Geometry check sheet. Reference: the model listing, model coordinates, mm. Round coordinates to 2 decimals unless told otherwise and drop trailing zeros. Write each loop counter-clockwise with the first axis right and the second up, starting at its lowest first coordinate (ties: lowest second). Pieces come first, ordered by that corner, then holes. Notation, with made-up numbers: (59.25, 6.25) - (92.25, 6.25) arc R21 ccw to (92.25, 32.25) - close; hole circle Ø4 at (15.5, 60). An arc over 180 degrees is marked (long way). Return JSON: item names as keys, results as strings.
```python
from build123d import *

# Parameters (mm, degrees)
SKETCH1_W           = 104
SKETCH1_H           = 104
SKETCH1_W_2         = 100
SKETCH1_H_2         = 100
BOSS_EXTRUDE1_DEPTH = 2


with BuildPart() as part:
    # Sketch1 → Boss-Extrude1 (new body)
    with BuildSketch(Plane(origin=(0, 0, 0), x_dir=(1, 0, 0), z_dir=(0, 1, 0))):
        Rectangle(SKETCH1_W, SKETCH1_H)
        Rectangle(SKETCH1_W_2, SKETCH1_H_2, mode=Mode.SUBTRACT)
    extrude(amount=BOSS_EXTRUDE1_DEPTH)


solid = part.part
```
(1) Section check B-B, the plane x = -30. Enter the section's corners in (y, z), plus the area to 3 significant figures.
Response values:
{"outline": "(0, -52) - (2, -52) - (2, -50) - (0, -50) - close; (0, 50) - (2, 50) - (2, 52) - (0, 52) - close", "area": "8.00 mm^2"}
(2) Section check A-A, the plane z = 21.5. Enter the section's corners in (x, y), plus the area to 3 significant figures.
Response values:
{"outline": "(-52, 0) - (-50, 0) - (-50, 2) - (-52, 2) - close; (50, 0) - (52, 0) - (52, 2) - (50, 2) - close", "area": "8.00 mm^2"}
(3) Section check C-C, the plane y = 1.45. Enter the section's corners in (x, z), plus the area to 3 significant figures.
Response values:
{"outline": "(-52, -52) - (52, -52) - (52, 52) - (-52, 52) - close; hole (-50, -50) - (50, -50) - (50, 50) - (-50, 50) - close", "area": "816 mm^2"}
(4) Material ranges on line 1 along Z through (x, y) = (-29.5, 0.9), recorded low to high. Write a range as [from, to].
Response values:
{"line 1": "z = [-52, -50], [50, 52]"}
